For this review, use the dimensioned drawing (mm, ordinates from the lowest corner) and the shaded views. A direction names the side the tool comes from. Coordinates: 2 decimals unless noted, no trailing zeros. Return JSON: item names as keys, results as strings. Group by question number.
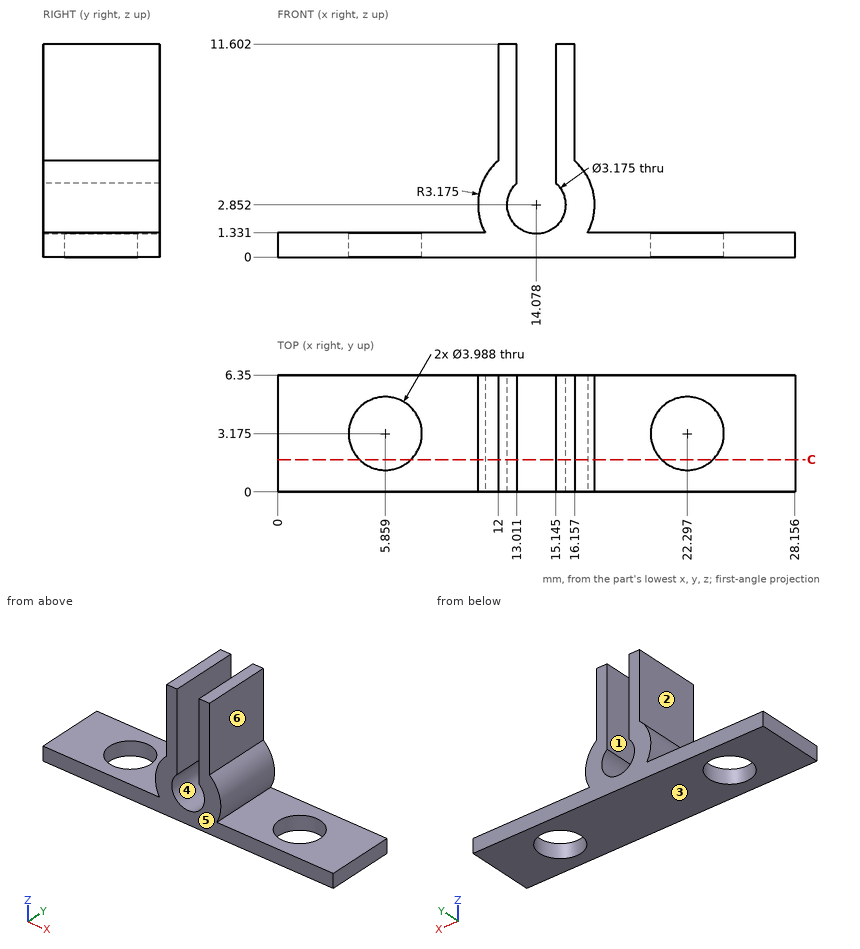
Item 1: Add section C-C (y = 1.75). Count the separate pieces of the cut face and the enclosed holes in it.
Item 2: The part is to be moulded in two halves that separate along X. For the marked faces 4, 5 and 6, say which applies: pulls with the +X half, pulls with the -X half, needs draft (parallel to the pull), parting line crosses it, or undercut.
Item 3: Machinability: for the marked faces 1, 2 and 3, which of the approach directions +Z, -Z, +X, -X, +Y, -Y give a long, thin tool a straight path to every point of the face, cutting with its end or side? Answer none if there is none.
Item 4: For pin 1 (1.9 mm diameter, centred on x = 14.08, z = 2.85, fed in from +Y); pin 2 (3 mm diameter, centred on y = 3, z = 8.5, fed in from -X); pin 3 (1 mm diameter, centred on y = 5.5, z = 8, fed in from +X), all flat-tipped, find the tip position at first contact; note any pin that passes through.
Item 5: For line 1 (X direction, y = 5.75, z = 5.5) (1 decimal); line 2 (X direction, y = 3.5, z = 1) (1 decimal); line 3 (X direction, y = 1.75, z = 4) (1 decimal), list the stretches that pass through material, from the lowest coordinate up.
Geometry check:
{
 "1": {"separate pieces": "3", "enclosed holes": "0"},
 "2": {"face 4": "undercut", "face 5": "needs draft", "face 6": "pulls with the +X half"},
 "3": {"face 1": "+Z, +Y, -Y", "face 2": "+Z, -X, +Y, -Y", "face 3": "-Z, +X, -X, +Y, -Y"},
 "4": {"pin 1": "through", "pin 2": "x = 12", "pin 3": "x = 16.16"},
 "5": {"line 1": "12 to 13, 15.1 to 16.2", "line 2": "0 to 3.9, 7.8 to 20.3, 24.3 to 28.2", "line 3": "11.1 to 13, 15.2 to 17"}
}
